Design review of the part built by this model. Coordinates are the model's own, in mm. Face numbers are marked on the shaded views. Coordinates: 2 decimals unless noted, no trailing zeros. Loops run counter-clockwise (first coordinate to the right, second up) from the corner with the lowest first, then second, coordinate; pieces in that order, holes last. Notation, with made-up numbers: (-12.75, -28) -> (37.25, -28) arc R29 cw to (37.25, 4) -> close; hole circle Ø5 at (59, 59.5). An arc over 180 degrees is marked (long way). Use one line per item in the form item = value. Start each with the question number.
1. Consider section A-A (z = 0). State the section outline as (x, y) points (3 decimals), then the cut area to 3 significant figures.
2. Consider section C-C (y = 0.4). State the section outline as (x, z) points (3 decimals).
3. Consider section D-D (z = 10.5). State the section outline as (x, y) points.
4. Consider section B-B (x = 0). State the section outline as (y, z) points (3 decimals).
5. The part is to be moulded in two halves that separate along Z. For the marked faces 1, 2 and 3, say which applies: released by +Z, released by -Z, zero draft, split by the parting line, or undercut.
6. For pin 1 (1 mm diameter, centred on x = 4.5, y = 0.5, fed in from +Z); pin 2 (1 mm diameter, centred on x = 7, y = 0.5, fed in from +Z), all flat-tipped, find the tip position at first contact; note any pin that passes through.
7. Wall thickness on line 1 (Z direction, x = -0.75, y = 1.1); line 2 (X direction, y = 0.25, z = -1.75); line 3 (X direction, y = 1.35, z = -10.5): over which ranges is each line inside the solid? List them lowest first. Write a range as from..to.
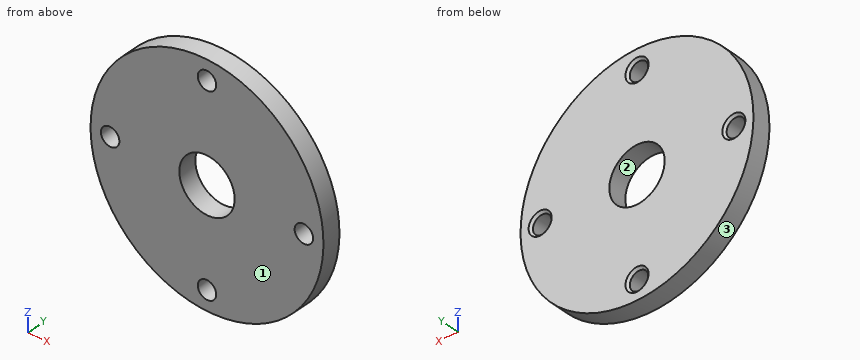
from build123d import *

# Parameters (mm, degrees)
SKETCH1_R             = 12.625
BOSS_EXTRUDE1_DEPTH   = 2
SKETCH2_R             = 0.5
CUT_EXTRUDE1_DEPTH    = 18.966113937
F_2_0MM_DOWEL_HOLE1_D = 2
CHAMFER1_SIZE         = 0.25
SKETCH4_R             = 3
CUT_EXTRUDE2_DEPTH    = 10


with BuildPart() as part:
    # Sketch1 → Boss-Extrude1 (new body)
    with BuildSketch(Plane(origin=(0, 0, 0), x_dir=(1, 0, 0), z_dir=(0, 1, 0))):
        with Locations(Location((0, 0, 0), (0, 0, 270))):
            Circle(SKETCH1_R)
    extrude(amount=BOSS_EXTRUDE1_DEPTH)

    # Sketch2 → Cut-Extrude1 (cut, through all)
    with BuildSketch(Plane(origin=(0, 2, 0), x_dir=(1, 0, 0), z_dir=(0, 1, 0))):
        with Locations(Location((0, 10.5, 0), (0, 0, 270))):
            Circle(SKETCH2_R)
        with Locations(Location((10.5, 0, 0), (0, 0, 270))):
            Circle(SKETCH2_R)
        with Locations(Location((0, -10.5, 0), (0, 0, 270))):
            Circle(SKETCH2_R)
        with Locations(Location((-10.5, 0, 0), (0, 0, 270))):
            Circle(SKETCH2_R)
    extrude(amount=-CUT_EXTRUDE1_DEPTH, mode=Mode.SUBTRACT)

    # Ø2.0mm Dowel Hole1 (through all)
    with Locations(Plane(origin=(-10.5, 2, 0), x_dir=(0, 0, 1), z_dir=(0, 1, 0))):
        with Locations((0, 0), (-10.5, 10.5), (0, 21), (10.5, 10.5)):
            Hole(F_2_0MM_DOWEL_HOLE1_D / 2)

    # Chamfer1
    chamfer1_edges = [part.edges().sort_by_distance(p)[0] for p in [
        (0, 2, 11.5),
        (10.5, 2, 1),
        (0, 2, -9.5),
        (-10.5, 2, 1),
    ]]
    chamfer(chamfer1_edges, length=CHAMFER1_SIZE)

    # Sketch4 → Cut-Extrude2 (cut)
    with BuildSketch(Plane(origin=(0, 2, 0), x_dir=(1, 0, 0), z_dir=(0, 1, 0))):
        with Locations(Location((0, 0, 0), (0, 0, 270))):
            Circle(SKETCH4_R)
    extrude(amount=-CUT_EXTRUDE2_DEPTH, mode=Mode.SUBTRACT)


solid = part.part
Geometry check:
q1.outline = (-12.625, 0) -> (-11.5, 0) -> (-11.5, 1.75) -> (-11.75, 2) -> (-12.625, 2) -> close; (-9.5, 0) -> (-3, 0) -> (-3, 2) -> (-9.25, 2) -> (-9.5, 1.75) -> close; (3, 0) -> (9.5, 0) -> (9.5, 1.75) -> (9.25, 2) -> (3, 2) -> close; (11.5, 0) -> (12.625, 0) -> (12.625, 2) -> (11.75, 2) -> (11.5, 1.75) -> close
q1.area = 30.4 mm²
q2.outline = circle Ø25.25 at (0, 0); hole circle Ø2 at (-10.5, 0); hole circle Ø6 at (0, 0); hole circle Ø2 at (0, -10.5); hole circle Ø2 at (0, 10.5); hole circle Ø2 at (10.5, 0)
q3.outline = (-7.01, 0) -> (-1, 0) -> (-1, 1.75) -> (-1.25, 2) -> (-7.01, 2) -> close; (1, 0) -> (7.01, 0) -> (7.01, 2) -> (1.25, 2) -> (1, 1.75) -> close
q4.outline = (0, -12.625) -> (2, -12.625) -> (2, -11.75) -> (1.75, -11.5) -> (0, -11.5) -> close; (0, -9.5) -> (1.75, -9.5) -> (2, -9.25) -> (2, -3) -> (0, -3) -> close; (0, 3) -> (2, 3) -> (2, 9.25) -> (1.75, 9.5) -> (0, 9.5) -> close; (0, 11.5) -> (1.75, 11.5) -> (2, 11.75) -> (2, 12.625) -> (0, 12.625) -> close
q5.face_1 = zero draft
q5.face_2 = undercut
q5.face_3 = split by the parting line
q6.pin_1 = 11.97
q6.pin_2 = 10.82
q7.line_1 = -12.6..-11.16, -9.84..-2.9, 2.9..9.84, 11.16..12.6
q7.line_2 = -12.5..-2.44, 2.44..12.5
q7.line_3 = -7.01..-1, 1..7.01
